```python
from build123d import *

# Parameters (mm, degrees)
BOSS_EXTRU_2_DEPTH      = 1
ESQUISSE2_OUTSIDE_W     = 37.018
ESQUISSE2_OUTSIDE_H     = 59.596
ENL_V_MAT_EXTRU_1_DEPTH = 27.837289407


with BuildPart() as part:
    # Esquisse1 → Boss.-Extru.2 (new body)
    with BuildSketch(Plane.XY):
        with BuildLine():
            Line((-12.922465041, 17.386083667), (-11.5420173, 16.419483753))
            ThreePointArc((-11.5420173, 16.419483753), (-8.998687611, 15.827772592), (-6.753604006, 17.161282102))
            ThreePointArc((-6.753604006, 17.161282102), (7.619740739, 15.766902052), (0, 3.5))
            ThreePointArc((0, 3.5), (-3.5, 0), (0, -3.5))
            ThreePointArc((0, -3.5), (7.619740739, -15.766902052), (-6.753604006, -17.161282102))
            ThreePointArc((-6.753604006, -17.161282102), (-8.998687611, -15.827772592), (-11.5420173, -16.419483753))
            Line((-11.5420173, -16.419483753), (-12.922465041, -17.386083667))
            ThreePointArc((-12.922465041, -17.386083667), (-12.266740841, -18.747374982), (-11.46812862, -20.030070109))
            Line((-11.46812862, -20.030070109), (-9.821287991, -18.876939886))
            ThreePointArc((-9.821287991, -18.876939886), (-9.457955178, -18.79240972), (-9.137228949, -18.982911079))
            ThreePointArc((-9.137228949, -18.982911079), (10.309061, -17.096396894), (0, -0.5))
            ThreePointArc((0, -0.5), (-0.5, 0), (0, 0.5))
            ThreePointArc((0, 0.5), (10.309061, 17.096396894), (-9.137228949, 18.982911079))
            ThreePointArc((-9.137228949, 18.982911079), (-9.457955178, 18.79240972), (-9.821287991, 18.876939886))
            Line((-9.821287991, 18.876939886), (-11.46812862, 20.030070109))
            ThreePointArc((-11.46812862, 20.030070109), (-12.266740841, 18.747374982), (-12.922465041, 17.386083667))
        make_face()
    extrude(amount=BOSS_EXTRU_2_DEPTH)

    # Esquisse2 outside → Enlèv. mat.-Extru.1 (cut, through all)
    with BuildSketch(Plane.XY.offset(1)):
        with Locations((-0.711, 0)):
            Rectangle(ESQUISSE2_OUTSIDE_W, ESQUISSE2_OUTSIDE_H)
        with BuildLine():
            Line((-12.922465041, 17.386083667), (-11.5420173, 16.419483753))
            ThreePointArc((-11.5420173, 16.419483753), (-8.998687611, 15.827772592), (-6.753604006, 17.161282102))
            ThreePointArc((-6.753604006, 17.161282102), (7.619740739, 15.766902052), (0, 3.5))
            ThreePointArc((0, 3.5), (-3.5, 0), (0, -3.5))
            ThreePointArc((0, -3.5), (7.619740739, -15.766902052), (-6.753604006, -17.161282102))
            ThreePointArc((-6.753604006, -17.161282102), (-8.998687611, -15.827772592), (-11.5420173, -16.419483753))
            Line((-11.5420173, -16.419483753), (-12.922465041, -17.386083667))
            Line((-12.922465041, -17.386083667), (-12.979954825, -18.647113037))
            Line((-12.979954825, -18.647113037), (-12.348888604, -18.205235712))
            Line((-12.348888604, -18.205235712), (-10.968440864, -17.238635798))
            ThreePointArc((-10.968440864, -17.238635798), (-9.1517768, -16.815984968), (-7.548145653, -17.768491761))
            ThreePointArc((-7.548145653, -17.768491761), (8.516180826, -16.210066999), (0, -2.5))
            ThreePointArc((0, -2.5), (-2.5, 0), (0, 2.5))
            ThreePointArc((0, 2.5), (8.516180826, 16.210066999), (-7.548145653, 17.768491761))
            ThreePointArc((-7.548145653, 17.768491761), (-9.1517768, 16.815984968), (-10.968440864, 17.238635798))
            Line((-10.968440864, 17.238635798), (-12.348888604, 18.205235712))
            Line((-12.348888604, 18.205235712), (-12.898926694, 18.590376529))
            Line((-12.898926694, 18.590376529), (-13.29562882, 18.205235712))
            Line((-13.29562882, 18.205235712), (-12.922465041, 17.386083667))
        make_face(mode=Mode.SUBTRACT)
    extrude(amount=-ENL_V_MAT_EXTRU_1_DEPTH, mode=Mode.SUBTRACT)


solid = part.part
```
Verification items for the finished model (mm, model axes). A direction names the side the tool comes from. Coordinates: 2 decimals unless noted, no trailing zeros. Write each loop counter-clockwise with the first axis right and the second up, starting at its lowest first coordinate (ties: lowest second). Pieces come first, ordered by that corner, then holes. Notation, with made-up numbers: M 68,30 L 109,30 A29 cw 109,53 Z; hole C -14.5,-35 d8. An arc over 180 degrees is marked long. One line per item, written item: value.
Item 1: Mould release check, pull along X, two halves, no side actions. Record for faces 4 (the flat face through (2, 3, 0)), 5 (the cylindrical face through (-9.13, 16.82, 0.51)), 6 (the cylindrical face through (-8.962, -15.834, 0.493)), 7 (the flat face through (-12.24, 16.91, 0.49)): pulls with the +X half, pulls with the -X half, needs draft (parallel to the pull), parting line crosses it, or undercut.
Check sheet entries:
face 4: needs draft
face 5: undercut
face 6: undercut
face 7: pulls with the -X half
Item 2: Section check B-B, the plane x = 2.5. Record the boundary of the cut face in (y, z), plus the area to 3 significant figures.
Check sheet entries:
outline: M -21.17,0 L -20.12,0 L -20.12,1 L -21.17,1 Z; M -3.88,0 L -2.83,0 L -2.83,1 L -3.88,1 Z; M 2.83,0 L 3.88,0 L 3.88,1 L 2.83,1 Z; M 20.12,0 L 21.17,0 L 21.17,1 L 20.12,1 Z
area: 4.16 mm^2
Item 3: Section check A-A, the plane z = 0.25. Record the boundary of the cut face in (x, y), plus the area to 3 significant figures.
Check sheet entries:
outline: M -12.92,-17.39 A14 ccw -12.5,-18.31 L -10.97,-17.24 A2.5 cw -7.55,-17.77 A9.5 ccw long 0,-2.5 A2.5 cw 0,2.5 A9.5 ccw long -7.55,17.77 A2.5 cw -10.97,17.24 L -12.5,18.31 A14 ccw -12.92,17.39 L -11.54,16.42 A3.5 ccw -6.75,17.16 A8.5 cw long 0,3.5 A3.5 ccw 0,-3.5 A8.5 cw long -6.75,-17.16 A3.5 ccw -11.54,-16.42 Z
area: 95.2 mm^2
Item 4: Section check D-D, the plane y = 12. Record the boundary of the cut face in (x, z).
Check sheet entries:
outline: M 8.5,0 L 9.5,0 L 9.5,1 L 8.5,1 Z
Item 5: Section check C-C, the plane x = -4.75. Record the boundary of the cut face in (y, z), plus the area to 3 significant figures.
Check sheet entries:
outline: M -20.23,0 L -19.05,0 L -19.05,1 L -20.23,1 Z; M 19.05,0 L 20.23,0 L 20.23,1 L 19.05,1 Z
area: 2.36 mm^2
Item 6: Access from +Z, -Z, +X, -X, +Y, -Y to the whole of each face (thin tool, end or side, straight path). Record for faces 1 (the flat face through (-12.223, -16.896, 0.493)), 2 (the cylindrical face through (-9.18, -16.81, 0.51)), 3 (the cylindrical face through (-9.04, 15.82, 0.49)).
Check sheet entries:
face 1: +Z, -Z, -X
face 2: +Z, -Z, -Y
face 3: +Z, -Z
Item 7: Scan lines: line 1 along X through (y, z) = (-18, 0.4); line 2 along Y through (x, z) = (0.75, 0.55); line 3 along Y through (x, z) = (7.25, 0.55). Record each from-to range of solid material in increasing order.
Check sheet entries:
line 1: x = -12.65 to -12.06, -7.37 to -6.02, 6.02 to 7.37
line 2: y = -21.47 to -20.47, -3.53 to -2.53, 2.53 to 3.53, 20.47 to 21.47
line 3: y = -18.14 to -16.44, -7.56 to -5.86, 5.86 to 7.56, 16.44 to 18.14
